```python
from build123d import *

# Parameters (mm, degrees)
SKETCH2_R                = 6.75
U_JOINT_BASE_DEPTH       = 3
U_JOINT_STANDUPS_DEPTH   = 9.5
STANDUP_ROUND_DEPTH      = 7.75
STANDUP_ROUND_DEPTH_BACK = 7.75
SKETCH5_R                = 1
BALL_HOLES_DEPTH         = 7.75
BALL_HOLES_DEPTH_BACK    = 7.75


with BuildPart() as part:
    # Sketch2 → U Joint Base (new body)
    with BuildSketch(Plane(origin=(0, 0, 0), x_dir=(-1, 0, 0), z_dir=(0, 0, -1))):
        Circle(SKETCH2_R)
    extrude(amount=U_JOINT_BASE_DEPTH)

    # Sketch3 → U Joint Standups (add)
    with BuildSketch(Plane(origin=(0, 0, -3), x_dir=(-1, 0, 0), z_dir=(0, 0, -1))):
        with BuildLine():
            Line((-5.771698, 3.5), (-3.75, 3.5))
            Line((-3.75, 3.5), (-3.75, -3.5))
            Line((-3.75, -3.5), (-5.771698, -3.5))
            ThreePointArc((-5.771698, -3.5), (-6.75, 0), (-5.771698, 3.5))
        make_face()
        with BuildLine():
            Line((3.75, -3.5), (3.75, 3.5))
            Line((3.75, 3.5), (5.771698, 3.5))
            ThreePointArc((5.771698, 3.5), (6.75, 0), (5.771698, -3.5))
            Line((5.771698, -3.5), (3.75, -3.5))
        make_face()
    extrude(amount=U_JOINT_STANDUPS_DEPTH)

    # Sketch4 → Standup Round (cut, two sides)
    with BuildSketch(Plane(origin=(0, 0, 0), x_dir=(0, 0, -1), z_dir=(1, 0, 0))) as standup_round_sk:
        with BuildLine():
            ThreePointArc((9, -3.5), (11.474874, -2.474874), (12.5, 0))
            Line((12.5, 0), (12.5, -3.5))
            Line((12.5, -3.5), (9, -3.5))
        make_face()
        with BuildLine():
            ThreePointArc((12.5, 0), (11.474874, 2.474874), (9, 3.5))
            Line((9, 3.5), (12.5, 3.5))
            Line((12.5, 3.5), (12.5, 0))
        make_face()
    extrude(amount=STANDUP_ROUND_DEPTH, mode=Mode.SUBTRACT)
    extrude(standup_round_sk.sketch, amount=-STANDUP_ROUND_DEPTH_BACK, mode=Mode.SUBTRACT)

    # Sketch5 → Ball Holes (cut, two sides)
    with BuildSketch(Plane(origin=(0, 0, 0), x_dir=(0, 0, -1), z_dir=(1, 0, 0))) as ball_holes_sk:
        with Locations((9, 0)):
            Circle(SKETCH5_R)
    extrude(amount=BALL_HOLES_DEPTH, mode=Mode.SUBTRACT)
    extrude(ball_holes_sk.sketch, amount=-BALL_HOLES_DEPTH_BACK, mode=Mode.SUBTRACT)


solid = part.part
```
Build history of the part. All positions in model axes, mm. A direction names the side the tool comes from. Give positions to 0.01 mm unless a question says otherwise; leave off trailing zeros. Loops run counter-clockwise (first coordinate to the right, second up) from the corner with the lowest first, then second, coordinate; pieces in that order, holes last. Notation, with made-up numbers: (23.5, 46) -> (52.5, 46) arc R24 cw to (52.5, 60) -> close; hole circle Ø10 at (75, 24). An arc over 180 degrees is marked (long way). One line per question, with ' | ' between items. Start each with the question number.
1) Cut at A-A (x = 4.75). Give the cut face in (y, z).
2) 3-axis set-ups, long thin cutter, end or side, ignore diameter. For faces 1 (the flat face through (5, -3.5, -6)), 2 (the flat face through (5, 3.5, -6)), 3 (the flat face through (3.75, 0, -7.7)): which of +Z, -Z, +X, -X, +Y, -Y reach the whole face in a straight line?
3) Probe L1, parallel to Z at x = 6.1, y = 0; L2, parallel to Y at x = 4.7, z = -9; L3, parallel to X at y = 0, z = -4.5. List the from-to ranges inside material, lowest first.
4) Cut at B-B (y = 1.5). Give the cut face in (x, z), plus the area to 3 significant figures.
5) Pin check, flat tips, straight feed: pin 1 (1 mm diameter, centred on x = -5, z = -6, fed in from -Y); pin 2 (2 mm diameter, centred on y = -2, z = -1.5, fed in from +X); pin 3 (0.6 mm diameter, centred on x = 5, z = -6.5, fed in from +Y). Stop position of each tip, or through.
6) Two-plate mould, pull along X, no slides. Class faces 4 (the flat face through (-3.75, 0, -7.7)), 5 (the flat face through (0, 0, 0)), 6 (the flat face through (0, 0, -3)): released by +X, released by -X, zero draft, split by the parting line, or undercut.
7) Cut at D-D (z = -1.5). Give the cut face in (x, y).
8) Cut at C-C (x = 0). Give the cut face in (y, z).
Return value:
1) outline: (-4.8, -3) -> (-3.5, -3) -> (-3.5, -9) arc R3.5 ccw to (0, -12.5) arc R3.5 ccw to (3.5, -9) -> (3.5, -3) -> (4.8, -3) -> (4.8, 0) -> (-4.8, 0) -> close; hole circle Ø2 at (0, -9)
2) face 1: -Z, +X, -X, -Y | face 2: -Z, +X, -X, +Y | face 3: -Z, +Y, -Y
3) L1: -12.5 to -10, -8 to 0 | L2: -3.5 to -1, 1 to 3.5 | L3: -6.75 to -3.75, 3.75 to 6.75
4) outline: (-6.58, -12.16) -> (-3.75, -12.16) -> (-3.75, -3) -> (3.75, -3) -> (3.75, -12.16) -> (6.58, -12.16) -> (6.58, 0) -> (-6.58, 0) -> close | area: 91.4 mm^2
5) pin 1: y = -3.5 | pin 2: x = 6.68 | pin 3: y = 3.5
6) face 4: undercut | face 5: zero draft | face 6: undercut
7) outline: circle Ø13.5 at (0, 0)
8) outline: (-6.75, -3) -> (6.75, -3) -> (6.75, 0) -> (-6.75, 0) -> close
